The listing builds one solid part. Answer for the finished solid, in the listing's coordinates (mm). Give positions to 0.01 mm unless a question says otherwise; leave off trailing zeros. Loops run counter-clockwise (first coordinate to the right, second up) from the corner with the lowest first, then second, coordinate; pieces in that order, holes last. Notation, with made-up numbers: (-32, 76) - (0, 76) arc R8 ccw to (0, 81) - close; hole circle Ø2 at (-24, -14.75). An arc over 180 degrees is marked (long way). Write item = value, one per line. Start each with the question number.
1) Consider probe 1 along Y at (x, z) = (2, -0.1); probe 2 along Y at (x, z) = (7.5, 0.6). Determine where each line is inside the solid, lowest interval first.
2) The part is cut by section B-B on z = 0.3. Write down the section's boundary in (x, y), plus the area to 3 significant figures.
3) The part is cut by section A-A on x = -6.25. Write down the section's boundary in (y, z).
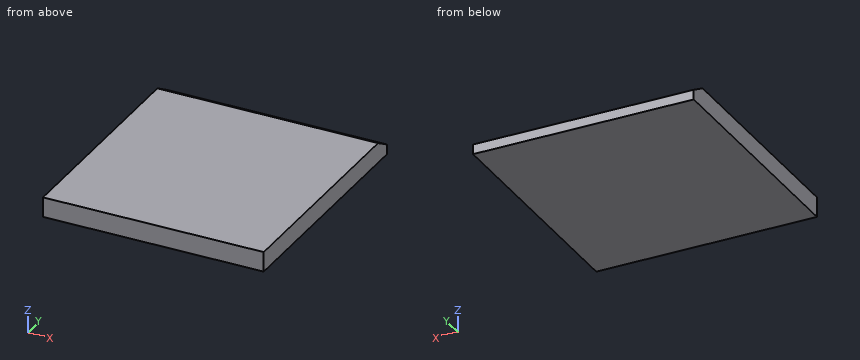
from build123d import *

# Parameters (mm, degrees)
F0_W     = 22.86
F0_H     = 2.54
F1_DEPTH = 24.638
F2_SIZE2 = 1.0265287786
F2_SIZE  = 1.778
F3_DEPTH = 0.508
F4_DEPTH = 0.1778
F5_DEPTH = 0.1778


with BuildPart() as f1:
    # F0 (on Front) → F1 (new body)
    with BuildSketch(Plane.XZ):
        Rectangle(F0_W, F0_H)
    extrude(amount=F1_DEPTH)

    # F2
    f2_edges = [f1.edges().sort_by_distance(p)[0] for p in [
        (0, 0, 1.27),
    ]]
    f2_side = f1.faces().sort_by_distance((0, -12.319, 1.27))[0]
    chamfer(f2_edges, length=F2_SIZE, length2=F2_SIZE2, reference=f2_side)

    # F3 (cut): faces of the model
    f3_faces = [f1.faces().sort_by_distance(p)[0] for p in [
        (0, -13.208, 1.27),
        (0, -0.889, 0.7567356107),
    ]]
    extrude(f3_faces, amount=-F3_DEPTH, dir=(0, 0, 1), mode=Mode.SUBTRACT)

    # F4 (cut): a face of the model
    f4_faces = [f1.faces().sort_by_distance(p)[0] for p in [
        (-11.43, -12.5367185417, -0.2665106389),
    ]]
    extrude(f4_faces, amount=-F4_DEPTH, mode=Mode.SUBTRACT)

    # F5 (cut): a face of the model
    f5_faces = [f1.faces().sort_by_distance(p)[0] for p in [
        (11.43, -12.5367185417, -0.2665106389),
    ]]
    extrude(f5_faces, amount=-F5_DEPTH, mode=Mode.SUBTRACT)


solid = f1.part
Answer below:
q1.probe_1 = -24.64 to -0.28
q1.probe_2 = -24.64 to -1.5
q2.outline = (-11.25, -24.64) - (11.25, -24.64) - (11.25, -0.98) - (-11.25, -0.98) - close
q2.area = 532 mm2
q3.outline = (-24.64, -1.27) - (0, -1.27) - (0, -0.26) - (-1.78, 0.76) - (-24.64, 0.76) - close
